Drawing for the job (mm, zero at the part's lowest x, y, z). A direction names the side the tool comes from. Round coordinates to 2 decimals unless told otherwise and drop trailing zeros. Order: outer loops, then holes, each group sorted by start corner. A loop starts at its lowest first (then second) coordinate and runs counter-clockwise, first axis right, second up. Notation, with made-up numbers: (-14, 27) -> (-7, 27) arc R23 cw to (-7, 37) -> close; hole circle Ø4 at (6, 4). An arc over 180 degrees is marked (long way). Use CSV: the item, a comma, the result in double quotes.
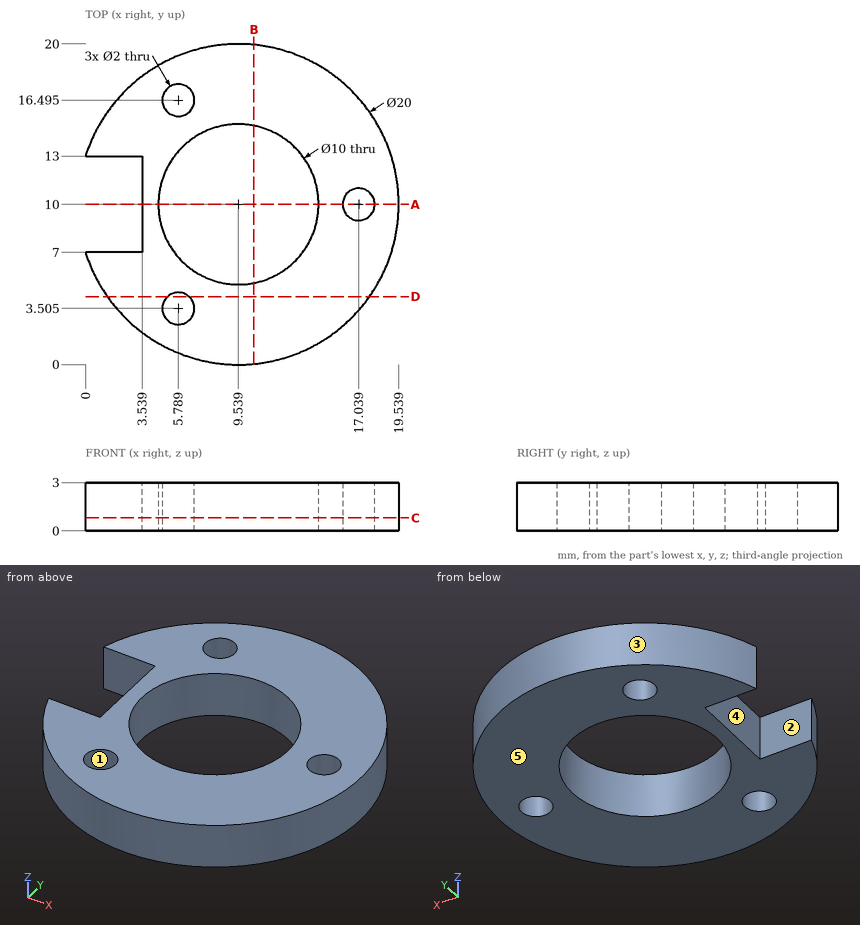
Q1. Which spindle directions (+Z, -Z, +X, -X, +Y, -Y) get a long thin tool onto all of the face, cutting with end or side? Do the marked faces 4 and 5. Say none if no direction does.
From the geometry:
face 4,"+Z, -Z, -X"
face 5,"-Z, +X, -X, +Y, -Y"
Q2. Mould opens along X. For the marked faces 1, 2 and 3 say: +X half, -X half, draft (parallel to the pull), parting line (faces both ways), or undercut.
From the geometry:
face 1,"undercut"
face 2,"draft"
face 3,"parting line"
Q3. Pin check, flat tips, straight feed: pin 1 (1.8 mm diameter, centred on x = 17.04, y = 10, fed in from -Z); pin 2 (1.5 mm diameter, centred on y = 13.5, z = 1, fed in from +X); pin 3 (1.5 mm diameter, centred on x = 1, z = 1.5, fed in from +Y); pin 4 (1.5 mm diameter, centred on x = 1, z = 2, fed in from -Y). Stop position of each tip, or through.
From the geometry:
pin 1,"passes through"
pin 2,"stops at x = 19.15"
pin 3,"stops at y = 16.27"
pin 4,"stops at y = 3.73"
Q4. Cut at A-A (y = 10). Give the cut face in (x, z), plus the area to 3 significant figures.
From the geometry:
outline,"(3.54, 0) -> (4.54, 0) -> (4.54, 3) -> (3.54, 3) -> close; (14.54, 0) -> (16.04, 0) -> (16.04, 3) -> (14.54, 3) -> close; (18.04, 0) -> (19.54, 0) -> (19.54, 3) -> (18.04, 3) -> close"
area,"12.0 mm²"
Q5. Cut at B-B (x = 10.5). Give the cut face in (y, z).
From the geometry:
outline,"(0.05, 0) -> (5.09, 0) -> (5.09, 3) -> (0.05, 3) -> close; (14.91, 0) -> (19.95, 0) -> (19.95, 3) -> (14.91, 3) -> close"
Q6. Cut at D-D (y = 4.25). Give the cut face in (x, z), plus the area to 3 significant figures.
From the geometry:
outline,"(1.36, 0) -> (5.12, 0) -> (5.12, 3) -> (1.36, 3) -> close; (6.46, 0) -> (17.72, 0) -> (17.72, 3) -> (6.46, 3) -> close"
area,"45.1 mm²"
Q7. Probe line 1 along X through (y, z) = (10, 1.5); line 2 along Y through (x, z) = (6.5, 2.5) (1 decimal); line 3 along X through (y, z) = (10.25, 0.45) (1 decimal). List the from-to ranges inside material, lowest first.
From the geometry:
line 1,"x = 3.54 to 4.54, 14.54 to 16.04, 18.04 to 19.54"
line 2,"y = 0.5 to 2.8, 4.2 to 6, 14 to 15.8, 17.2 to 19.5"
line 3,"x = 3.5 to 4.5, 14.5 to 16.1, 18 to 19.5"
Q8. Cut at C-C (z = 0.8). Give the cut face in (x, y) (1 decimal), plus the area to 3 significant figures.
From the geometry:
outline,"(0, 7) arc R10 ccw (long way) to (0, 13) -> (3.5, 13) -> (3.5, 7) -> close; hole circle Ø10 at (9.5, 10); hole circle Ø2 at (5.8, 3.5); hole circle Ø2 at (5.8, 16.5); hole circle Ø2 at (17, 10)"
area,"203 mm²"
